Input: part model. Units: mm. Frame: model coordinates. A direction names the side the tool comes from. Give positions to 0.01 mm unless a question says otherwise; leave off trailing zeros. Loops run counter-clockwise (first coordinate to the right, second up) from the corner with the lowest first, then second, coordinate; pieces in that order, holes last. Notation, with made-up numbers: (40, 20) - (68, 20) arc R15 ccw to (68, 30) - close; hole circle Ø3 at (-38, 62.5). An arc over 180 degrees is marked (long way). Answer as a JSON object with one key per item and string values. Group by question number.
(1) Mould query, pull axis X, two halves, no side actions, for faces 1 (the flat face through (12.7, 0, 2)), 2 (the flat face through (10.16, 0, -2)), 3 (the flat face through (0.1, -25.4, 2.4)). Classes: +X half, -X half, draft (parallel to the pull), parting line (faces both ways), or undercut.
(2) Section query B-B (z = 94.5). Return loops of the section in (x, y), plus the area to 3 significant figures.
(3) Access query for faces 4 (the flat face through (-12.7, 0, 2)), 5 (the flat face through (0.1, -22.86, -2.4)). Directions: +Z, -Z, +X, -X, +Y, -Y. A direction counts if a zero-diameter tool reaches every point of the face in a straight line with its end or side. Return the directions, or none.
(4) Section query A-A (y = 15.5). Return loops of the section in (x, z).
(5) Material intervals for L1, parallel to Y at x = -8.5, z = -21; L2, parallel to X at y = -19, z = -63; L3, parallel to X at y = 23.45, z = 101.6, sorted ascending.
```python
from build123d import *

# Parameters (mm, degrees)
SKETCH1_W                 = 342.9
SKETCH1_H                 = 50.8
BOSS_EXTRUDE1_DEPTH       = 25.4
SKETCH2_W                 = 20.32
SKETCH2_H                 = 45.72
CUT_EXTRUDE1_DEPTH        = 343.9
F_6_CLEARANCE_HOLE1_D     = 4.1402
F_6_CLEARANCE_HOLE1_DEPTH = 50.8
F_6_CLEARANCE_HOLE2_D     = 4.1402
F_6_CLEARANCE_HOLE2_DEPTH = 50.8
FILLET1_R                 = 0.5
FILLET2_R                 = 2.54


with BuildPart() as part:
    # Sketch1 → Boss-Extrude1 (new body)
    with BuildSketch(Plane(origin=(12.7, 0, 0), x_dir=(0, 0, -1), z_dir=(1, 0, 0))):
        Rectangle(SKETCH1_W, SKETCH1_H)
    extrude(amount=-BOSS_EXTRUDE1_DEPTH)

    # Sketch2 → Cut-Extrude1 (cut, through all)
    with BuildSketch(Plane(origin=(0, 0, -171.45), x_dir=(-1, 0, 0), z_dir=(0, 0, -1))):
        Rectangle(SKETCH2_W, SKETCH2_H)
    extrude(amount=-CUT_EXTRUDE1_DEPTH, mode=Mode.SUBTRACT)

    # #6 Clearance Hole1
    with Locations(Plane(origin=(0, -25.4, 0), x_dir=(-1, 0, 0), z_dir=(0, -1, 0))):
        with Locations((0, 711.2), (0, 736.6), (0, 685.8), (0, 660.4), (0, 635), (0, 609.6), (0, 584.2), (0, 558.8), (0, 533.4), (0, 508), (0, 482.6), (0, 457.2), (0, 431.8), (0, 406.4), (0, 381), (0, 355.6), (0, 330.2), (0, 304.8), (0, 279.4), (0, 254), (0, 228.6), (0, 203.2), (0, 177.8), (0, 152.4), (0, 127), (0, 101.6), (0, 76.2), (0, 50.8), (0, 25.4), (0, 0), (0, -25.4), (0, -50.8), (0, -76.2), (0, -101.6), (0, -127), (0, -152.4), (0, -177.8), (0, -203.2), (0, -228.6), (0, -254), (0, -279.4), (0, -304.8), (0, -330.2), (0, -355.6), (0, -381), (0, -406.4), (0, -431.8), (0, -457.2), (0, -482.6), (0, -508), (0, -533.4), (0, -558.8), (0, -584.2), (0, -609.6), (0, -635), (0, -660.4), (0, -685.8), (0, -711.2), (0, -736.6)):
            Hole(F_6_CLEARANCE_HOLE1_D / 2, depth=F_6_CLEARANCE_HOLE1_DEPTH)

    # #6 Clearance Hole2
    with Locations(Plane(origin=(0, 25.4, 0), x_dir=(1, 0, 0), z_dir=(0, 1, 0))):
        with Locations((0, 711.2), (0, 736.6), (0, 685.8), (0, 660.4), (0, 635), (0, 609.6), (0, 584.2), (0, 558.8), (0, 533.4), (0, 508), (0, 482.6), (0, 457.2), (0, 431.8), (0, 406.4), (0, 381), (0, 355.6), (0, 330.2), (0, 304.8), (0, 279.4), (0, 254), (0, 228.6), (0, 203.2), (0, 177.8), (0, 152.4), (0, 127), (0, 101.6), (0, 76.2), (0, 50.8), (0, 25.4), (0, 0), (0, -25.4), (0, -50.8), (0, -76.2), (0, -101.6), (0, -127), (0, -152.4), (0, -177.8), (0, -203.2), (0, -228.6), (0, -254), (0, -279.4), (0, -304.8), (0, -330.2), (0, -355.6), (0, -381), (0, -406.4), (0, -431.8), (0, -457.2), (0, -482.6), (0, -508), (0, -533.4), (0, -558.8), (0, -584.2), (0, -609.6), (0, -635), (0, -660.4), (0, -685.8), (0, -711.2), (0, -736.6)):
            Hole(F_6_CLEARANCE_HOLE2_D / 2, depth=F_6_CLEARANCE_HOLE2_DEPTH)

    # Fillet1
    fillet1_edges = [part.edges().sort_by_distance(p)[0] for p in [
        (-10.16, -22.86, 0),
        (10.16, -22.86, 0),
        (10.16, 22.86, 0),
        (-10.16, 22.86, 0),
    ]]
    fillet(fillet1_edges, radius=FILLET1_R)

    # Fillet2
    fillet2_edges = [part.edges().sort_by_distance(p)[0] for p in [
        (-12.7, 25.4, 0),
        (-12.7, -25.4, 0),
        (12.7, 25.4, 0),
        (12.7, -25.4, 0),
    ]]
    fillet(fillet2_edges, radius=FILLET2_R)


solid = part.part
```
Recorded:
{
 "1": {"face 1": "+X half", "face 2": "undercut", "face 3": "draft"},
 "2": {"outline": "(-12.7, -22.86) arc R2.54 ccw to (-10.16, -25.4) - (10.16, -25.4) arc R2.54 ccw to (12.7, -22.86) - (12.7, 22.86) arc R2.54 ccw to (10.16, 25.4) - (-10.16, 25.4) arc R2.54 ccw to (-12.7, 22.86) - close; hole (-10.16, -22.36) arc R0.5 ccw to (-9.66, -22.86) - (9.66, -22.86) arc R0.5 ccw to (10.16, -22.36) - (10.16, 22.36) arc R0.5 ccw to (9.66, 22.86) - (-9.66, 22.86) arc R0.5 ccw to (-10.16, 22.36) - close", "area": "356 mm^2"},
 "3": {"face 4": "+Z, -Z, -X, +Y, -Y", "face 5": "+Z, -Z"},
 "4": {"outline": "(-12.7, -171.45) - (-10.16, -171.45) - (-10.16, 171.45) - (-12.7, 171.45) - close; (10.16, -171.45) - (12.7, -171.45) - (12.7, 171.45) - (10.16, 171.45) - close"},
 "5": {"L1": "y = -25.4 to -22.86, 22.86 to 25.4", "L2": "x = -12.7 to -10.16, 10.16 to 12.7", "L3": "x = -12.63 to -2.07, 2.07 to 12.63"}
}
